from build123d import *

# Parameters (mm, degrees)
SKIZZE1_R                       = 12.25
AUFSATZ_LINEAR_AUSTRAGEN1_DEPTH = 13
VERRUNDUNG1_R                   = 5
WANDUNG1_T                      = -1.6
FASE1_SIZE                      = 0.5


with BuildPart() as part:
    # Skizze1 → Aufsatz-Linear austragen1 (new body)
    with BuildSketch(Plane(origin=(0, 0, 0), x_dir=(1, 0, 0), z_dir=(0, 1, 0))):
        with Locations(Location((0, 0, 0), (0, 0, 90))):
            Circle(SKIZZE1_R)
    extrude(amount=AUFSATZ_LINEAR_AUSTRAGEN1_DEPTH)

    # Verrundung1
    verrundung1_edges = [part.edges().sort_by_distance(p)[0] for p in [
        (0, 0, 12.25),
    ]]
    fillet(verrundung1_edges, radius=VERRUNDUNG1_R)

    # Wandung1
    wandung1_openings = [part.faces().sort_by_distance(p)[0] for p in [
        (0, 13, 0),
    ]]
    offset(amount=WANDUNG1_T, openings=wandung1_openings, kind=Kind.INTERSECTION)

    # Fase1
    fase1_edges = [part.edges().sort_by_distance(p)[0] for p in [
        (0, 13, 12.25),
        (0, 13, 10.65),
    ]]
    chamfer(fase1_edges, length=FASE1_SIZE)


solid = part.part
For this review, take the finished solid that the model builds, in its own axes (mm). A direction names the side the tool comes from. Give positions to 0.01 mm unless a question says otherwise; leave off trailing zeros. Order: outer loops, then holes, each group sorted by start corner. A loop starts at its lowest first (then second) coordinate and runs counter-clockwise, first axis right, second up. Notation, with made-up numbers: M 77.5,75.5 L 122.5,75.5 A7 cw 122.5,84.5 Z; hole C -17.5,23.5 d4. An arc over 180 degrees is marked long. Answer in a Markdown table with one row per item. Add a question column.
(1) Consider section B-B on z = 0. State the section outline as (x, y) points, and give its area (3 significant figures).
(2) For pin 1 (5 mm diameter, centred on x = -6.5, y = 5, fed in from +Z); pin 2 (1.5 mm diameter, centred on y = 7, z = -6.5, fed in from +X); pin 3 (4 mm diameter, centred on x = 9.5, z = -4.5, fed in from -Y), all flat-tipped, find the tip position at first contact; note any pin that passes through.
(3) For faces 4 (the face through (0, 0, 0)), 5 (the face through (0, 1.6, 0)), list the 3-axis set-ups (+Z, -Z, +X, -X, +Y, -Y) from which the entire face can be reached by the end or side of a thin tool; tool diameter is ignored.
(4) Consider section A-A on x = 0. State the section outline as (y, z) points.
(5) Consider section C-C on y = 9. State the section outline as (x, z) points, and give its area (3 significant figures).
(6) Mouldability with a two-part tool opening along X and no side actions: class faces 1 (the face through (-8.98, 8.698, -5.725)), 2 (the face through (-3.68, 8.698, -11.684)), 3 (the face through (7, 13, 9)) as +X half, -X half, draft (parallel to the pull), parting line (faces both ways), or undercut.
(7) Wall thickness on probe 1 along X at (y, z) = (8, 0); probe 2 along Y at (x, z) = (1.25, 3.75); probe 3 along X at (y, z) = (6, -3.75): over which ranges is each line inside the solid? List them lowest first. Write a range as [from, to].
Evaluation:
| question | item | result |
|---|---|---|
| 1 | outline | M -12.25,5 A5 ccw -7.25,0 L 7.25,0 A5 ccw 12.25,5 L 12.25,12.5 L 11.75,13 L 11.15,13 L 10.65,12.5 L 10.65,5 A3.4 cw 7.25,1.6 L -7.25,1.6 A3.4 cw -10.65,5 L -10.65,12.5 L -11.15,13 L -11.75,13 L -12.25,12.5 Z |
| 1 | area | 69.4 mm^2 |
| 2 | pin 1 | stops at z = 11.58 |
| 2 | pin 2 | stops at x = 10.82 |
| 2 | pin 3 | stops at y = 0.16 |
| 3 | face 4 | +Z, -Z, +X, -X, -Y |
| 3 | face 5 | +Y |
| 4 | outline | M 0,-7.25 A5 ccw 5,-12.25 L 12.5,-12.25 L 13,-11.75 L 13,-11.15 L 12.5,-10.65 L 5,-10.65 A3.4 cw 1.6,-7.25 L 1.6,7.25 A3.4 cw 5,10.65 L 12.5,10.65 L 13,11.15 L 13,11.75 L 12.5,12.25 L 5,12.25 A5 ccw 0,7.25 Z |
| 5 | outline | C 0,0 d24.5; hole C 0,0 d21.3 |
| 5 | area | 115 mm^2 |
| 6 | face 1 | undercut |
| 6 | face 2 | parting line |
| 6 | face 3 | draft |
| 7 | probe 1 | x = [-12.25, -10.65], [10.65, 12.25] |
| 7 | probe 2 | y = [0, 1.6] |
| 7 | probe 3 | x = [-11.66, -9.97], [9.97, 11.66] |
